The listing builds one solid part. Answer for the finished solid, in the listing's coordinates (mm). Round coordinates to 2 decimals unless told otherwise and drop trailing zeros. Loops run counter-clockwise (first coordinate to the right, second up) from the corner with the lowest first, then second, coordinate; pieces in that order, holes last. Notation, with made-up numbers: (47.25, -27.75) - (91.25, -27.75) arc R22 cw to (91.25, -7.75) - close; hole circle Ø6 at (-10.75, -16). An arc over 180 degrees is marked (long way). Write item = value, one per line. Start each with the question number.
1) Section A-A, the plane z = 0 is taken. Determine the outline of the cut face in (x, y).
2) Section D-D, the plane z = -13 is taken. Determine the outline of the cut face in (x, y), and give its area (3 significant figures).
3) Section C-C, the plane y = -1.85 is taken. Give the number of separate pieces and of enclosed holes in the cut face, and give its area (3 significant figures).
4) For a pull along Z with two mould halves and no side action, classify faces 1 (the flat face through (-25.4, -2, 0)), 2 (the cylindrical face through (-18.513, -2.348, 23.096)), 3 (the cylindrical face through (82.1, -2.35, -29.44)) as released by +Z, released by -Z, zero draft, split by the parting line, or undercut.
5) Section B-B, the plane x = 61 is taken. Determine the outline of the cut face in (y, z).
6) Straight lines are drawn through the part: line 1 along Z through (x, y) = (0, -2.4); line 2 along Z through (x, y) = (-19, -1.9); line 3 along Z through (x, y) = (60.96, -1.25). For each, find the intervals that lie inside material, in ascending order.
7) Given pin 1 Ø3 at (x, z) = (78.1, 25.35) entering from +Y, flat-ended and moving along its own axis, determine where the tip first touches the part or whether it passes through.
from build123d import *

# Parameters (mm, degrees)
F0_R     = 2.54
F0_R_2   = 2.4892
F0_R_3   = 9.5885
F0_R_4   = 14.2621
F1_DEPTH = 4.7625


# Not quite as in the source:
# - a length typed as a fraction of an inch, garbled in the dataset ("3 / 203.2 mm" for 3/8 in), is restored


with BuildPart() as f1:
    # F0 (on Front) → F1 (new body)
    with BuildSketch(Plane.XZ):
        with BuildLine():
            Line((83.82, -25.3516301214), (83.82, 25.3492))
            ThreePointArc((83.82, 25.3492), (82.1461152545, 29.3903152545), (78.105, 31.0642))
            Line((78.105, 31.0642), (-19.685, 31.0642))
            ThreePointArc((-19.685, 31.0642), (-23.7261152545, 29.3903152545), (-25.4, 25.3492))
            Line((-25.4, 25.3492), (-25.4, -25.3516301214))
            ThreePointArc((-25.4, -25.3516301214), (-23.7915717475, -29.3262110405), (-19.8716383264, -31.0635817261))
            Line((-19.8716383264, -31.0635817261), (-19.4987171118, -31.063593329))
            Line((-19.4987171118, -31.063593329), (78.1048221862, -31.0666301186))
            ThreePointArc((78.1048221862, -31.0666301186), (82.1460523873, -29.392808242), (83.82, -25.3516301214))
        make_face()
        with Locations((-19.685, -25.3516301214)):
            Circle(F0_R, mode=Mode.SUBTRACT)
        with Locations((0, -25.4)):
            Circle(F0_R_2, mode=Mode.SUBTRACT)
        with Locations((78.105, -25.3516301214)):
            Circle(F0_R, mode=Mode.SUBTRACT)
        Circle(F0_R_3, mode=Mode.SUBTRACT)
        with Locations((-19.685, 25.3492)):
            Circle(F0_R, mode=Mode.SUBTRACT)
        with Locations((0, 25.4)):
            Circle(F0_R_2, mode=Mode.SUBTRACT)
        with Locations((30.48, 0)):
            Circle(F0_R_4, mode=Mode.SUBTRACT)
        with Locations((60.96, 0)):
            Circle(F0_R_4, mode=Mode.SUBTRACT)
        with Locations((78.105, 25.3492)):
            Circle(F0_R, mode=Mode.SUBTRACT)
        with BuildLine():
            ThreePointArc((-19.8716383264, -31.0635817261), (-19.6851778138, -31.0666301186), (-19.4987171118, -31.063593329))
            Line((-19.4987171118, -31.063593329), (-19.8716383264, -31.0635817261))
        make_face()
    extrude(amount=F1_DEPTH)


solid = f1.part
Geometry check:
q1.outline = (-25.4, -4.76) - (-9.59, -4.76) - (-9.59, 0) - (-25.4, 0) - close; (9.59, -4.76) - (16.22, -4.76) - (16.22, 0) - (9.59, 0) - close; (44.74, -4.76) - (46.7, -4.76) - (46.7, 0) - (44.74, 0) - close; (75.22, -4.76) - (83.82, -4.76) - (83.82, 0) - (75.22, 0) - close
q2.outline = (-25.4, -4.76) - (24.61, -4.76) - (24.61, 0) - (-25.4, 0) - close; (36.35, -4.76) - (55.09, -4.76) - (55.09, 0) - (36.35, 0) - close; (66.83, -4.76) - (83.82, -4.76) - (83.82, 0) - (66.83, 0) - close
q2.area = 408 mm2
q3.separate_pieces = 1
q3.enclosed_holes = 9
q3.area = 5,070 mm2
q4.face_1 = zero draft
q4.face_2 = undercut
q4.face_3 = released by -Z
q5.outline = (-4.76, -31.07) - (0, -31.07) - (0, -14.26) - (-4.76, -14.26) - close; (-4.76, 14.26) - (0, 14.26) - (0, 31.06) - (-4.76, 31.06) - close
q6.line_1 = -31.06 to -27.89, -22.91 to -9.59, 9.59 to 22.91, 27.89 to 31.06
q6.line_2 = -31.06 to -27.8, -22.91 to 22.9, 27.8 to 31.06
q6.line_3 = -31.07 to -14.26, 14.26 to 31.06
q7.pin_1 = through
